Part model, mm, in its own coordinate system. A direction names the side the tool comes from. Round coordinates to 2 decimals unless told otherwise and drop trailing zeros. Loops run counter-clockwise (first coordinate to the right, second up) from the corner with the lowest first, then second, coordinate; pieces in that order, holes last. Notation, with made-up numbers: M -13.5,-2.5 L 38.5,-2.5 A21 cw 38.5,20.5 Z; hole C -24.5,24 d3. An arc over 180 degrees is marked long. Put each result on its own line as item: value. Start each with the question number.
1) Which spindle directions (+Z, -Z, +X, -X, +Y, -Y) get a long thin tool onto all of the face, cutting with end or side? Do faces 5 (the flat face through (-141, 15, 8)), 6 (the flat face through (-148, 110, 10)), 7 (the flat face through (-76, 110, 0)), 8 (the flat face through (-3, 109, 10)). Say none if no direction does.
2) Probe line 1 along Y through (x, z) = (-100, 1.25); line 2 along Y through (x, z) = (-20.5, 4.5); line 3 along X through (y, z) = (116.5, 7). List the from-to ranges inside material, lowest first.
3) Slice it at A-A on x = -105. Give the cut face in (y, z).
4) Slice it at B-B on y = 96. Give the cut face in (x, z), then the cut area to 3 significant figures.
5) Pull direction Y, two halves, no side cores. Call faces 1 (the flat face through (-76, 0, 5)), 2 (the flat face through (-145, 110, 6)), 3 (the flat face through (-76, 217, 5)), 4 (the flat face through (-143, 210, 13)): +Y half, -Y half, draft (parallel to the pull), parting line (faces both ways), or undercut.
6) Drop flat-ended pins along their axis: pin 1 Ø1.3 at (x, y) = (-25, 4) entering from -Z; pin 2 Ø2 at (x, y) = (-95, 5) entering from +Z; pin 3 Ø2.5 at (x, y) = (-30, 150) entering from +Z; pin 4 Ø0.9 at (x, y) = (-95, 4.5) entering from -Z. Give the stop position or say it passes through.
```python
from build123d import *

# Parameters (mm, degrees)
SKETCH_W        = 150
SKETCH_H        = 217
SKETCH_R        = 1.15
SKETCH_R_2      = 1.75
PAD_DEPTH       = 3
SKETCH001_W     = 150
SKETCH001_H     = 217
PAD001_DEPTH    = 7
SKETCH002_R     = 1.75
SKETCH002_R_2   = 1
POCKET_DEPTH    = 5
SKETCH003_R     = 1.15
POCKET001_DEPTH = 7.5
SKETCH004_R     = 1.15
POCKET002_DEPTH = 10
SKETCH005_W     = 15
SKETCH005_H     = 15
PAD002_DEPTH    = 3


with BuildPart() as part:
    # Sketch → Pad (new body)
    with BuildSketch(Plane.XY):
        with Locations((-75, 108.5)):
            Rectangle(SKETCH_W, SKETCH_H)
        with Locations((-140, 40)):
            Circle(SKETCH_R, mode=Mode.SUBTRACT)
        with Locations((-130, 40)):
            Circle(SKETCH_R, mode=Mode.SUBTRACT)
        with Locations((-120, 40)):
            Circle(SKETCH_R, mode=Mode.SUBTRACT)
        with Locations((-110, 40)):
            Circle(SKETCH_R, mode=Mode.SUBTRACT)
        with Locations((-100, 40)):
            Circle(SKETCH_R, mode=Mode.SUBTRACT)
        with Locations((-90, 40)):
            Circle(SKETCH_R, mode=Mode.SUBTRACT)
        with Locations((-80, 40)):
            Circle(SKETCH_R, mode=Mode.SUBTRACT)
        with Locations((-70, 40)):
            Circle(SKETCH_R, mode=Mode.SUBTRACT)
        with Locations((-60, 40)):
            Circle(SKETCH_R, mode=Mode.SUBTRACT)
        with Locations((-50, 40)):
            Circle(SKETCH_R, mode=Mode.SUBTRACT)
        with Locations((-40, 40)):
            Circle(SKETCH_R, mode=Mode.SUBTRACT)
        with Locations((-30, 40)):
            Circle(SKETCH_R, mode=Mode.SUBTRACT)
        with Locations((-20, 40)):
            Circle(SKETCH_R, mode=Mode.SUBTRACT)
        with Locations((-10, 40)):
            Circle(SKETCH_R, mode=Mode.SUBTRACT)
        with Locations((-140, 50)):
            Circle(SKETCH_R, mode=Mode.SUBTRACT)
        with Locations((-130, 50)):
            Circle(SKETCH_R, mode=Mode.SUBTRACT)
        with Locations((-120, 50)):
            Circle(SKETCH_R, mode=Mode.SUBTRACT)
        with Locations((-110, 50)):
            Circle(SKETCH_R, mode=Mode.SUBTRACT)
        with Locations((-100, 50)):
            Circle(SKETCH_R, mode=Mode.SUBTRACT)
        with Locations((-90, 50)):
            Circle(SKETCH_R, mode=Mode.SUBTRACT)
        with Locations((-80, 50)):
            Circle(SKETCH_R, mode=Mode.SUBTRACT)
        with Locations((-70, 50)):
            Circle(SKETCH_R, mode=Mode.SUBTRACT)
        with Locations((-60, 50)):
            Circle(SKETCH_R, mode=Mode.SUBTRACT)
        with Locations((-50, 50)):
            Circle(SKETCH_R, mode=Mode.SUBTRACT)
        with Locations((-40, 50)):
            Circle(SKETCH_R, mode=Mode.SUBTRACT)
        with Locations((-30, 50)):
            Circle(SKETCH_R, mode=Mode.SUBTRACT)
        with Locations((-20, 50)):
            Circle(SKETCH_R, mode=Mode.SUBTRACT)
        with Locations((-10, 50)):
            Circle(SKETCH_R, mode=Mode.SUBTRACT)
        with Locations((-140, 140)):
            Circle(SKETCH_R, mode=Mode.SUBTRACT)
        with Locations((-130, 140)):
            Circle(SKETCH_R, mode=Mode.SUBTRACT)
        with Locations((-120, 140)):
            Circle(SKETCH_R, mode=Mode.SUBTRACT)
        with Locations((-110, 140)):
            Circle(SKETCH_R, mode=Mode.SUBTRACT)
        with Locations((-100, 140)):
            Circle(SKETCH_R, mode=Mode.SUBTRACT)
        with Locations((-90, 140)):
            Circle(SKETCH_R, mode=Mode.SUBTRACT)
        with Locations((-80, 140)):
            Circle(SKETCH_R, mode=Mode.SUBTRACT)
        with Locations((-70, 140)):
            Circle(SKETCH_R, mode=Mode.SUBTRACT)
        with Locations((-60, 140)):
            Circle(SKETCH_R, mode=Mode.SUBTRACT)
        with Locations((-50, 140)):
            Circle(SKETCH_R, mode=Mode.SUBTRACT)
        with Locations((-40, 140)):
            Circle(SKETCH_R, mode=Mode.SUBTRACT)
        with Locations((-30, 140)):
            Circle(SKETCH_R, mode=Mode.SUBTRACT)
        with Locations((-20, 140)):
            Circle(SKETCH_R, mode=Mode.SUBTRACT)
        with Locations((-10, 140)):
            Circle(SKETCH_R, mode=Mode.SUBTRACT)
        with Locations((-140, 150)):
            Circle(SKETCH_R, mode=Mode.SUBTRACT)
        with Locations((-130, 150)):
            Circle(SKETCH_R, mode=Mode.SUBTRACT)
        with Locations((-120, 150)):
            Circle(SKETCH_R, mode=Mode.SUBTRACT)
        with Locations((-110, 150)):
            Circle(SKETCH_R, mode=Mode.SUBTRACT)
        with Locations((-100, 150)):
            Circle(SKETCH_R, mode=Mode.SUBTRACT)
        with Locations((-90, 150)):
            Circle(SKETCH_R, mode=Mode.SUBTRACT)
        with Locations((-80, 150)):
            Circle(SKETCH_R, mode=Mode.SUBTRACT)
        with Locations((-70, 150)):
            Circle(SKETCH_R, mode=Mode.SUBTRACT)
        with Locations((-60, 150)):
            Circle(SKETCH_R, mode=Mode.SUBTRACT)
        with Locations((-50, 150)):
            Circle(SKETCH_R, mode=Mode.SUBTRACT)
        with Locations((-40, 150)):
            Circle(SKETCH_R, mode=Mode.SUBTRACT)
        with Locations((-30, 150)):
            Circle(SKETCH_R, mode=Mode.SUBTRACT)
        with Locations((-20, 150)):
            Circle(SKETCH_R, mode=Mode.SUBTRACT)
        with Locations((-10, 150)):
            Circle(SKETCH_R, mode=Mode.SUBTRACT)
        with Locations((-125, 209)):
            Circle(SKETCH_R_2, mode=Mode.SUBTRACT)
        with Locations((-55, 209)):
            Circle(SKETCH_R_2, mode=Mode.SUBTRACT)
        with Locations((-125, 5)):
            Circle(SKETCH_R, mode=Mode.SUBTRACT)
        with Locations((-55, 5)):
            Circle(SKETCH_R, mode=Mode.SUBTRACT)
        with Locations((-25, 5)):
            Circle(SKETCH_R, mode=Mode.SUBTRACT)
        with Locations((-95, 5)):
            Circle(SKETCH_R, mode=Mode.SUBTRACT)
        with Locations((-25, 209)):
            Circle(SKETCH_R_2, mode=Mode.SUBTRACT)
        with Locations((-95, 209)):
            Circle(SKETCH_R_2, mode=Mode.SUBTRACT)
    extrude(amount=PAD_DEPTH)

    # Sketch001 → Pad001 (join)
    with BuildSketch(Plane.XY.offset(3)):
        with Locations((-75, 108.5)):
            Rectangle(SKETCH001_W, SKETCH001_H)
        Polygon((-5, 212), (-135, 212), (-135, 202), (-145, 202), (-145, 15), (-135, 15), (-135, 5), (-5, 5), align=None, mode=Mode.SUBTRACT)
    extrude(amount=PAD001_DEPTH)

    # Sketch002 → Pocket (cut)
    with BuildSketch(Plane.YZ):
        with Locations((17, 6.5)):
            Circle(SKETCH002_R)
        with Locations((107, 6.5)):
            Circle(SKETCH002_R)
        with Locations((197, 6.5)):
            Circle(SKETCH002_R)
        with Locations((10, 6.5)):
            Circle(SKETCH002_R_2)
        with Locations((210, 6.5)):
            Circle(SKETCH002_R_2)
    extrude(amount=-POCKET_DEPTH, mode=Mode.SUBTRACT)

    # Sketch003 → Pocket001 (cut, symmetric)
    with BuildSketch(Plane.YZ.offset(-150)):
        with Locations((107, 6.5)):
            Circle(SKETCH003_R)
        with Locations((17, 6.5)):
            Circle(SKETCH003_R)
        with Locations((197, 6.5)):
            Circle(SKETCH003_R)
    extrude(amount=POCKET001_DEPTH, both=True, mode=Mode.SUBTRACT)

    # Sketch004 → Pocket002 (cut)
    with BuildSketch(Plane.XZ):
        with Locations((-4, 6)):
            Circle(SKETCH004_R)
        with Locations((-146, 6)):
            Circle(SKETCH004_R)
    extrude(amount=-POCKET002_DEPTH, mode=Mode.SUBTRACT)

    # Sketch005 → Pad002 (join)
    with BuildSketch(Plane.XY.offset(10)):
        with Locations((-142.5, 209.5)):
            Rectangle(SKETCH005_W, SKETCH005_H)
        with Locations((-142.5, 7.5)):
            Rectangle(SKETCH005_W, SKETCH005_H)
    extrude(amount=PAD002_DEPTH)


solid = part.part
```
Recorded:
1. face 5: +Z
1. face 6: +Z, +X, -X
1. face 7: -Z, +X, -X, +Y, -Y
1. face 8: +Z, +X, +Y, -Y
2. line 1: y = 0 to 38.85, 41.15 to 48.85, 51.15 to 138.85, 141.15 to 148.85, 151.15 to 217
2. line 2: y = 0 to 5, 212 to 217
2. line 3: x = -150 to -145, -5 to 0
3. outline: M 0,0 L 217,0 L 217,10 L 212,10 L 212,3 L 5,3 L 5,10 L 0,10 Z
4. outline: M -150,0 L 0,0 L 0,10 L -5,10 L -5,3 L -145,3 L -145,10 L -150,10 Z
4. area: 520 mm2
5. face 1: -Y half
5. face 2: undercut
5. face 3: +Y half
5. face 4: draft
6. pin 1: stops at z = 0
6. pin 2: stops at z = 10
6. pin 3: stops at z = 3
6. pin 4: stops at z = 3
